Here's how the part is built. I have some questions about the finished solid (model axes, mm). A direction names the side the tool comes from. Coordinates: 2 decimals unless noted, no trailing zeros. Write each loop counter-clockwise with the first axis right and the second up, starting at its lowest first coordinate (ties: lowest second). Pieces come first, ordered by that corner, then holes. Notation, with made-up numbers: M 43,-25.75 L 95,-25.75 A17 ccw 95,-19.75 Z; hole C -35,53 d2. An arc over 180 degrees is marked long. Use a Markdown table: item, result.
```python
from build123d import *

# Parameters (mm, degrees)
BOSS_EXTRUDE1_DEPTH = 50.8
SKETCH2_W           = 7.239
SKETCH2_H           = 3.81
BOSS_EXTRUDE2_DEPTH = 63.5
RIB1_START          = -1.27
RIB1_DEPTH          = 2.54
FILLET1_R           = 2.54


# Read off the part's stored shape, not the designer's step: Rib1
with BuildPart() as part:
    # Sketch1 → Boss-Extrude1 (new body)
    with BuildSketch(Plane.XY):
        Polygon((3.6195, -31.75), (0, -31.75), (-3.6195, -31.75), (-3.6195, -33.02), (-4.8895, -33.02), (-4.8895, -34.29), (-4.8895, -40.259), (4.8895, -40.259), (4.8895, -34.29), (4.8895, -33.02), (3.6195, -33.02), align=None)
        Polygon((-4.8895, -40.259), (-4.8895, -34.29), (-7.474152818, -35.78225), align=None)
        Polygon((7.474152818, -35.78225), (4.8895, -34.29), (4.8895, -40.259), align=None)
        Polygon((-3.6195, 33.02), (-3.6195, 31.75), (0, 31.75), (3.6195, 31.75), (3.6195, 33.02), (4.8895, 33.02), (4.8895, 34.29), (4.8895, 40.259), (-4.8895, 40.259), (-4.8895, 34.29), (-4.8895, 33.02), align=None)
        Polygon((-7.474152818, 35.78225), (-4.8895, 34.29), (-4.8895, 40.259), align=None)
        Polygon((7.474152818, 35.78225), (4.8895, 40.259), (4.8895, 34.29), align=None)
    extrude(amount=-BOSS_EXTRUDE1_DEPTH)

    # Sketch2 → Boss-Extrude2 (add)
    with BuildSketch(Plane.XZ.offset(-31.75)):
        with Locations((0, -1.905)):
            Rectangle(SKETCH2_W, SKETCH2_H)
    extrude(amount=BOSS_EXTRUDE2_DEPTH)

    # Rib1 outline → Rib1 (add)
    with BuildSketch(Plane(origin=(0, 0, 0), x_dir=(0, 0, -1), z_dir=(1, 0, 0)).offset(RIB1_START)):
        with BuildLine():
            ThreePointArc((33.02, -31.75), (21.87573729, 0), (33.02, 31.75))
            Line((33.02, 31.75), (3.81, 31.75))
            Line((3.81, 31.75), (3.81, -31.75))
            Line((3.81, -31.75), (33.02, -31.75))
        make_face()
    extrude(amount=RIB1_DEPTH)

    # Fillet1
    # the kernel refuses this fillet: 2.54 mm, written as the material it adds along each edge
    with BuildSketch(Plane(origin=(-1.27, 31.75, -39.352115439), x_dir=(-1, 0, 0), z_dir=(0, 0, 1))) as fillet1_piece_1_section:
        with BuildLine():
            CenterArc((2.54, 2.532846176), FILLET1_R, 180, 85.698777695)
            Line((0, 2.532846176), (0, 0))
            Line((0, 0), (2.3495, 0))
        make_face()
    fillet1_piece_1 = extrude(amount=35.542115439, mode=Mode.PRIVATE)
    fillet1_piece_1 = fillet1_piece_1 - Plane(origin=(-1.944090085, 0, -72.675737291), x_dir=(0, -0.6249999999925505, 0.7806247498057642), z_dir=(-1, 0, 0)) * Cylinder(50.800000001, 82, mode=Mode.PRIVATE)
    add(fillet1_piece_1)
    with BuildSketch(Plane(origin=(-1.27, 38.082115439, -3.81), x_dir=(-1, 0, 0), z_dir=(0, -1, 0))) as fillet1_piece_2:
        with BuildLine():
            CenterArc((2.54, 2.532846176), FILLET1_R, 180, 85.698777695)
            Line((0, 2.532846176), (0, 0))
            Line((0, 0), (2.3495, 0))
        make_face()
    extrude(amount=76.164230879)
    with BuildSketch(Plane(origin=(-1.27, -31.75, -3.81), x_dir=(-1, 0, 0), z_dir=(0, 0, -1))) as fillet1_piece_3_section:
        with BuildLine():
            CenterArc((2.54, 2.532846176), FILLET1_R, 180, 85.698777695)
            Line((0, 2.532846176), (0, 0))
            Line((0, 0), (2.3495, 0))
        make_face()
    fillet1_piece_3 = extrude(amount=35.542115439, mode=Mode.PRIVATE)
    fillet1_piece_3 = fillet1_piece_3 - Plane(origin=(-1.944090085, 0, -72.675737291), x_dir=(0, -0.6249999999925505, 0.7806247498057642), z_dir=(-1, 0, 0)) * Cylinder(50.800000001, 82, mode=Mode.PRIVATE)
    add(fillet1_piece_3)
    with BuildSketch(Plane(origin=(1.27, 31.75, -39.352115439), x_dir=(1, 0, 0), z_dir=(0, 0, 1))) as fillet1_piece_4_section:
        with BuildLine():
            CenterArc((2.54, -2.532846176), FILLET1_R, 94.301222305, 85.698777695)
            Line((0, -2.532846176), (0, 0))
            Line((0, 0), (2.3495, 0))
        make_face()
    fillet1_piece_4 = extrude(amount=35.542115439, mode=Mode.PRIVATE)
    fillet1_piece_4 = fillet1_piece_4 - Plane(origin=(1.944090085, 0, -72.675737291), x_dir=(0, -0.6249999999925505, 0.7806247498057642), z_dir=(-1, 0, 0)) * Cylinder(50.800000001, 82, mode=Mode.PRIVATE)
    add(fillet1_piece_4)
    with BuildSketch(Plane(origin=(1.27, -31.75, -3.81), x_dir=(1, 0, 0), z_dir=(0, 0, -1))) as fillet1_piece_5_section:
        with BuildLine():
            CenterArc((2.54, -2.532846176), FILLET1_R, 94.301222305, 85.698777695)
            Line((0, -2.532846176), (0, 0))
            Line((0, 0), (2.3495, 0))
        make_face()
    fillet1_piece_5 = extrude(amount=35.542115439, mode=Mode.PRIVATE)
    fillet1_piece_5 = fillet1_piece_5 - Plane(origin=(1.944090085, 0, -72.675737291), x_dir=(0, -0.6249999999925505, 0.7806247498057642), z_dir=(-1, 0, 0)) * Cylinder(50.800000001, 82, mode=Mode.PRIVATE)
    add(fillet1_piece_5)
    with BuildSketch(Plane(origin=(1.27, 38.082115439, -3.81), x_dir=(0, 0, -1), z_dir=(0, -1, 0))) as fillet1_piece_6:
        with BuildLine():
            CenterArc((2.532846176, 2.54), FILLET1_R, 184.301222305, 85.698777695)
            Line((0, 2.3495), (0, 0))
            Line((0, 0), (2.532846176, 0))
        make_face()
    extrude(amount=76.164230879)


solid = part.part
```
1. I need wall thicknesses on probe 1 along Y at (x, z) = (-3.5, -8); probe 2 along Y at (x, z) = (-6, -27); probe 3 along X at (y, z) = (25, -21). Which ranges of each line are inside material? Lowest first, please.
Answers follow:
| item | result |
|---|---|
| probe 1 | y = -40.26 to -31.74, 31.74 to 40.26 |
| probe 2 | y = -38.34 to -34.93, 34.93 to 38.34 |
| probe 3 | x = -1.27 to 1.27 |
2. Suppose I cut it at A-A on z = -37.5. Write out the boundary of the cut face in (x, y).
Answers follow:
| item | result |
|---|---|
| outline | M -7.47,-35.78 L -4.89,-40.26 L 4.89,-40.26 L 7.47,-35.78 L 4.89,-34.29 L 4.89,-33.02 L 3.62,-33.02 L 3.62,-31.75 L -3.62,-31.75 L -3.62,-33.02 L -4.89,-33.02 L -4.89,-34.29 Z; M -7.47,35.78 L -4.89,34.29 L -4.89,33.02 L -3.62,33.02 L -3.62,31.75 L 3.62,31.75 L 3.62,33.02 L 4.89,33.02 L 4.89,34.29 L 7.47,35.78 L 4.89,40.26 L -4.89,40.26 Z |
3. Suppose I cut it at C-C on x = -6. Write out the boundary of the cut face in (y, z), and give its area (3 significant figures).
Answers follow:
| item | result |
|---|---|
| outline | M -38.34,-50.8 L -34.93,-50.8 L -34.93,0 L -38.34,0 Z; M 34.93,-50.8 L 38.34,-50.8 L 38.34,0 L 34.93,0 Z |
| area | 346 mm2 |
4. Will these pins go through, and if not, where does the flat tip stop? pin 1 Ø12 at (y, z) = (21, -8.5) entering from -X; pin 2 Ø1.5 at (x, y) = (2, 0) entering from +Z; pin 3 Ø8 at (x, y) = (-2, 16.5) entering from -Z; pin 4 Ø1.4 at (y, z) = (33.5, -15.5) entering from -X.
Answers follow:
| item | result |
|---|---|
| pin 1 | stops at x = -3.62 |
| pin 2 | stops at z = 0 |
| pin 3 | stops at z = -26.17 |
| pin 4 | stops at x = -4.89 |
5. Which directions (+Z, -Z, +X, -X, +Y, -Y) give clear straight access to the entire face, cutting with the end or side of a thin tool? Please do faces 1 (the face through (-6.164, -35.026, -25.044)), 2 (the face through (6.2, -35.047, -25.044)), 3 (the face through (2, -31, -18)).
Answers follow:
| item | result |
|---|---|
| face 1 | +Z, -Z, -X |
| face 2 | +Z, -Z, +X |
| face 3 | -Z, +X |
6. Suppose I cut it at D-D on y = 13.5. Write out the boundary of the cut face in (x, z), and give its area (3 significant figures).
Answers follow:
| item | result |
|---|---|
| outline | M -3.62,-3.81 A2.54 cw -1.27,-6.34 L -1.27,-23.7 L 1.27,-23.7 L 1.27,-6.34 A2.54 cw 3.62,-3.81 L 3.62,0 L -3.62,0 Z |
| area | 80.8 mm2 |
7. Suppose I cut it at B-B on x = -0.25. Write out the boundary of the cut face in (y, z), and give its area (3 significant figures).
Answers follow:
| item | result |
|---|---|
| outline | M -40.26,-50.8 L -31.75,-50.8 L -31.75,-33.02 A50.8 cw 31.75,-33.02 L 31.75,-50.8 L 40.26,-50.8 L 40.26,0 L -40.26,0 Z |
| area | 2,480 mm2 |
